Design review of the part built by this model. Coordinates are the model's own, in mm. A direction names the side the tool comes from. Coordinates: 2 decimals unless noted, no trailing zeros. Loops run counter-clockwise (first coordinate to the right, second up) from the corner with the lowest first, then second, coordinate; pieces in that order, holes last. Notation, with made-up numbers: M 14,31 L 43,31 A20 cw 43,65 Z; hole C 88,-40 d1. An arc over 180 degrees is marked long. Answer as a JSON object with one key per item and string values. Group by question number.
1. Consider section B-B (x = 22.5). State the section outline as (y, z) points.
2. Consider section C-C (y = -23). State the section outline as (x, z) points.
3. Consider section D-D (z = 23.5). State the section outline as (x, y) points.
4. Insertion check: pin 1 (8 mm diameter, centred on x = 56.5, z = 14.5, fed in from +Y); pin 2 (0.8 mm diameter, centred on x = 5, z = 39.5, fed in from +Y); pin 3 (2.5 mm diameter, centred on x = 22.5, y = -14, fed in from +Z). Each pin has a flat end and moves straight along its axis. Give the tip position at first contact, or say it passes through.
5. Machinability: for faces 5 (the flat face through (15, -17, 4)), 6 (the flat face through (11.3, -14, 42.2)), 7 (the flat face through (10, -16, 40.7)), 8 (the flat face through (43, -27, 21)), which of the approach directions +Z, -Z, +X, -X, +Y, -Y give a long, thin tool a straight path to every point of the face, cutting with its end or side? Answer none if there is none.
6. Draft analysis for pull direction X (two halves, no side actions). For faces 1 (the cylindrical face through (11.63, -21.32, -0.49)), 2 (the cylindrical face through (12.82, -9.57, 1.54)), 3 (the cylindrical face through (56.617, -26.479, 10.398)), 4 (the flat face through (7.7, -16.2, 44.2)), state which applies: +X half, -X half, draft (parallel to the pull), parting line (faces both ways), or undercut.
7. Consider section A-A (z = 31.6). State the section outline as (x, y) points.
8. To check wall thickness, follow probe 1 along X at (y, z) = (-26.35, 10.6); probe 2 along Z at (x, y) = (8, -12.5); probe 3 along Z at (x, y) = (6.5, -2.5). State the ranges of each line that lie inside material, in increasing order.
from build123d import *

# Parameters (mm, degrees)
PERFIL_LATERAL_DEPTH        = 42.2
SKETCH7_W                   = 40
SKETCH7_H                   = 34.2
CORTE_VERTICAL_PERFIL_DEPTH = 84.191586113
SKETCH8_R                   = 6
SOPORTE_AL_EJE_GIRO_1_DEPTH = 2
SKETCH10_R                  = 7.5
SOPORTE_AL_EJE_GIRO_2_DEPTH = 1
SKETCH11_R                  = 5.25
EJE_GIRO_DEPTH              = 5
SERVO_HORN_BED_DEPTH        = 2.5
SKETCH13_R                  = 1.55
HUECOS_BASE_LASER_DEPTH     = 83.230408001
FILLET1_R                   = 8
DECORACION_START            = 1
SKETCH14_R                  = 7.5
DECORACION_HORN_DEPTH       = 1
SKETCH15_R                  = 5
DECORACION_HORN_2_DEPTH     = 1
TORNILLOS_HORN_DEPTH        = 85.22374962
TORNILLOS_HORN_DEPTH_BACK   = 1.5
SKETCH12_R                  = 1.15
SKETCH12_R_2                = 1
SKETCH16_R                  = 3
CABEZA_TORNILLO_HORN_DEPTH  = 2
SKETCH17_W                  = 12
SKETCH17_H                  = 11
CUT_EXTRUDE9_DEPTH          = 2
FILLET2_R                   = 2


with BuildPart() as part:
    # Sketch6 → Perfil lateral (new body)
    with BuildSketch(Plane.XY):
        Polygon((0, 0), (15, 0), (40, -25), (66, -25), (66, -28), (0, -28), align=None)
    extrude(amount=PERFIL_LATERAL_DEPTH)

    # Sketch7 → Corte vertical perfil (cut, through all)
    with BuildSketch(Plane(origin=(0, 0, 0), x_dir=(1, 0, 0), z_dir=(0, 1, 0))):
        with Locations((20, -21.1)):
            Rectangle(SKETCH7_W, SKETCH7_H)
    extrude(amount=-CORTE_VERTICAL_PERFIL_DEPTH, mode=Mode.SUBTRACT)

    # Sketch8 → soporte al eje giro 1 (add)
    with BuildSketch(Plane.XY):
        with Locations((10, -14)):
            Circle(SKETCH8_R)
    extrude(amount=-SOPORTE_AL_EJE_GIRO_1_DEPTH)

    # Sketch10 → soporte al eje giro 2 (add)
    with BuildSketch(Plane(origin=(0, 0, 0), x_dir=(-1, 0, 0), z_dir=(0, 0, -1))):
        with Locations((-10, -14)):
            Circle(SKETCH10_R)
    extrude(amount=SOPORTE_AL_EJE_GIRO_2_DEPTH)

    # Sketch11 → eje giro (cut)
    with BuildSketch(Plane.XY.offset(4)):
        with Locations((10, -14)):
            Circle(SKETCH11_R)
    extrude(amount=-EJE_GIRO_DEPTH, mode=Mode.SUBTRACT)

    # Sketch9 → servo horn bed (cut)
    with BuildSketch(Plane.XY.offset(38.2)):
        with BuildLine():
            Line((0, -17.7), (10, -17.7))
            Line((10, -17.7), (25, -16.012614746))
            ThreePointArc((25, -16.012614746), (27, -14), (25, -11.987385254))
            Line((25, -11.987385254), (10, -10.3))
            Line((10, -10.3), (0, -10.3))
            Line((0, -10.3), (0, -17.7))
        make_face()
    extrude(amount=SERVO_HORN_BED_DEPTH, mode=Mode.SUBTRACT)

    # Sketch13 → Huecos base laser (cut, through all)
    with BuildSketch(Plane(origin=(0, -25, 0), x_dir=(1, 0, 0), z_dir=(0, 1, 0))):
        with Locations(Location((55.079807472, -31.6, 0), (0, 0, 270))):
            Circle(SKETCH13_R)
        with Locations(Location((42.529807472, -31.6, 0), (0, 0, 270))):
            Circle(SKETCH13_R)
        with Locations(Location((42.529807472, -10.6, 0), (0, 0, 270))):
            Circle(SKETCH13_R)
        with Locations(Location((55.079807472, -10.6, 0), (0, 0, 270))):
            Circle(SKETCH13_R)
    extrude(amount=-HUECOS_BASE_LASER_DEPTH, mode=Mode.SUBTRACT)

    # Fillet1
    fillet1_edges = [part.edges().sort_by_distance(p)[0] for p in [
        (0, 0, 40.2),
        (15, 0, 40.2),
        (0, -28, 40.2),
        (0, 0, 2),
        (15, 0, 2),
        (0, -28, 2),
    ]]
    fillet(fillet1_edges, radius=FILLET1_R)

    # Sketch14 → Decoracion horn (add)
    with BuildSketch(Plane.XY.offset(42.2).offset(DECORACION_START)):
        with Locations(Location((10, -14, 0), (0, 0, 180))):
            Circle(SKETCH14_R)
    extrude(amount=-DECORACION_HORN_DEPTH)

    # Sketch15 → Decoracion Horn 2 (add)
    with BuildSketch(Plane.XY.offset(43.2)):
        with Locations((10, -14)):
            Circle(SKETCH15_R)
    extrude(amount=DECORACION_HORN_2_DEPTH)

    # Sketch12 → Tornillos horn (cut, two sides: drawn at the far end of the back side and taken through both)
    with BuildSketch(Plane.XY.offset(42.2).offset(-TORNILLOS_HORN_DEPTH_BACK)):
        with Locations((10, -14)):
            Circle(SKETCH12_R)
        with Locations(Location((15, -14, 0), (0, 0, 264.260829523))):
            Circle(SKETCH12_R_2)
        with Locations(Location((19, -14, 0), (0, 0, 180))):
            Circle(SKETCH12_R_2)
        with Locations(Location((22.5, -14, 0), (0, 0, 180))):
            Circle(SKETCH12_R_2)
    extrude(amount=TORNILLOS_HORN_DEPTH + TORNILLOS_HORN_DEPTH_BACK, mode=Mode.SUBTRACT)

    # Sketch16 → cabeza tornillo horn (cut)
    with BuildSketch(Plane.XY.offset(44.2)):
        with Locations((10, -14)):
            Circle(SKETCH16_R)
    extrude(amount=-CABEZA_TORNILLO_HORN_DEPTH, mode=Mode.SUBTRACT)

    # Sketch17 → Cut-Extrude9 (cut)
    with BuildSketch(Plane(origin=(0, -25, 0), x_dir=(1, 0, 0), z_dir=(0, 1, 0))):
        with Locations((40, -21.1)):
            Rectangle(SKETCH17_W, SKETCH17_H)
    extrude(amount=-CUT_EXTRUDE9_DEPTH, mode=Mode.SUBTRACT)

    # Fillet2
    fillet2_edges = [part.edges().sort_by_distance(p)[0] for p in [
        (66, -26.5, 42.2),
        (66, -26.5, 0),
    ]]
    fillet(fillet2_edges, radius=FILLET2_R)


solid = part.part
Findings below:
{
 "1": {"outline": "M -28,0 L -7.5,0 L -7.5,4 L -28,4 Z; M -28,38.2 L -16.29,38.2 L -16.29,40.7 L -15,40.7 L -15,42.2 L -28,42.2 Z; M -13,40.7 L -11.71,40.7 L -11.71,38.2 L -7.5,38.2 L -7.5,42.2 L -13,42.2 Z"},
 "2": {"outline": "M 0.58,0 L 38,0 L 38,4 L 0.58,4 Z; M 0.58,38.2 L 38,38.2 L 38,42.2 L 0.58,42.2 Z"},
 "3": {"outline": "M 40,-28 L 66,-28 L 66,-25 L 46,-25 L 46,-27 L 40,-27 Z"},
 "4": {"pin 1": "stops at y = -25", "pin 2": "stops at y = -0.43", "pin 3": "stops at z = 42.2"},
 "5": {"face 5": "-X, +Y, -Y", "face 6": "+Z", "face 7": "-X", "face 8": "-X, +Y"},
 "6": {"face 1": "parting line", "face 2": "undercut", "face 3": "undercut", "face 4": "draft"},
 "7": {"outline": "M 40,-28 L 40.98,-28 L 40.98,-25 L 40,-25 Z; M 44.08,-28 L 53.53,-28 L 53.53,-25 L 44.08,-25 Z; M 56.63,-28 L 66,-28 L 66,-25 L 56.63,-25 Z"},
 "8": {"probe 1": "x = 40 to 40.98, 44.08 to 53.53, 56.63 to 66", "probe 2": "z = -2 to -1, 40.7 to 42.2", "probe 3": "z = 0 to 4, 38.2 to 42.2"}
}
